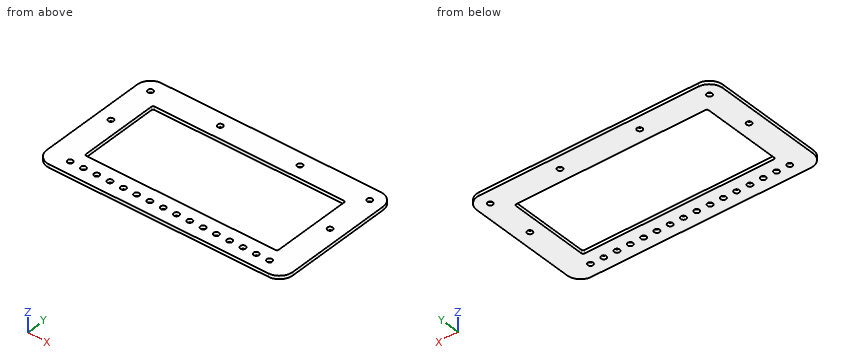
Autodesk Inventor part; units mm, degrees
ref_plane "YZ Plane" through (0, 0, 0) normal (1, 0, 0) x (0, 1, 0)
ref_plane "XZ Plane" through (0, 0, 0) normal (0, 1, 0) x (-1, 0, 0)
ref_plane "XY Plane" through (0, 0, 0) normal (0, 0, 1) x (1, 0, 0)
sketch "Sketch1" plane through (0, 0, 0) normal (0, 0, 1) x (1, 0, 0)
  line L0 (-92.075, -39.37) -> (92.075, -39.37)
  line L1 (92.075, -39.37) -> (92.075, 39.37)
  line L2 (92.075, 39.37) -> (-92.075, 39.37)
  line L3 (-92.075, 39.37) -> (-92.075, -39.37)
  line L4 (-92.075, -39.37) -> (92.075, 39.37) construction
  line L5 (92.075, -39.37) -> (-92.075, 39.37) construction
  line L6 (-117.475, 64.77) -> (117.475, 64.77)
  line L7 (117.475, 64.77) -> (117.475, -64.77)
  line L8 (117.475, -64.77) -> (-117.475, -64.77)
  line L9 (-117.475, -64.77) -> (-117.475, 64.77)
  point P0 (0, 0)
  dimension "d0" = 184.15
  dimension "d1" = 78.74
  dimension "d2" = 25.4
extrude "Plate1" add sketch "Sketch1" along normal mid plane 3.175
sketch "Sketch2" plane through (0, 0, 1.5875) normal (0, 0, 1) x (1, 0, 0)
  line L0 (-92.075, -39.37) -> (-92.075, 39.37) construction
  line L1 (-92.075, 39.37) -> (92.075, 39.37) construction
  line L2 (92.075, 39.37) -> (92.075, -39.37) construction
  line L3 (92.075, -39.37) -> (-92.075, -39.37) construction
  line L4 (104.775, 52.07) -> (-104.775, 52.07) construction
  line L5 (-104.775, 52.07) -> (-104.775, -52.07) construction
  line L6 (-104.775, -52.07) -> (104.775, -52.07) construction
  line L7 (104.775, -52.07) -> (104.775, 52.07) construction
  line L8 (0, 90.678) -> (0, -90.678) construction
  point P0 (0, 0)
  point P1 (-95.25, -52.07)
  point P2 (-82.55, -52.07)
  point P3 (-69.85, -52.07)
  point P4 (-57.15, -52.07)
  point P5 (-44.45, -52.07)
  point P6 (-31.75, -52.07)
  point P7 (-19.05, -52.07)
  point P8 (-6.35, -52.07)
  point P9 (6.35, -52.07)
  point P10 (19.05, -52.07)
  point P11 (31.75, -52.07)
  point P12 (44.45, -52.07)
  point P13 (57.15, -52.07)
  point P14 (69.85, -52.07)
  point P15 (82.55, -52.07)
  point P16 (95.25, -52.07)
  point P17 (-38.1, 52.07)
  point P18 (38.1, 52.07)
  point P19 (-104.775, 6.35)
  point P20 (104.775, 6.35)
  dimension "d4" = 12.7
  dimension "d16" = 12.7
  dimension "d21" = 9.525
  dimension "d22" = 9.525
  dimension "d23" = 66.675
  dimension "d24" = 66.675
  dimension "d25" = 76.2
  dimension "d26" = 45.72
  dimension "d28" = 45.72
hole "Hole1" at (-104.775, 52.07, 1.5875) at (104.775, 52.07, 1.5875) at (-95.25, -52.07, 1.5875) at (-82.55, -52.07, 1.5875) at (-69.85, -52.07, 1.5875) at (-57.15, -52.07, 1.5875) at (-44.45, -52.07, 1.5875) at (-31.75, -52.07, 1.5875) at (-19.05, -52.07, 1.5875) at (-6.35, -52.07, 1.5875) at (6.35, -52.07, 1.5875) at (19.05, -52.07, 1.5875) at (31.75, -52.07, 1.5875) at (44.45, -52.07, 1.5875) at (57.15, -52.07, 1.5875) at (69.85, -52.07, 1.5875) at (82.55, -52.07, 1.5875) at (95.25, -52.07, 1.5875) at (-38.1, 52.07, 1.5875) at (38.1, 52.07, 1.5875) at (-104.775, 6.35, 1.5875) at (104.775, 6.35, 1.5875) direction (0, 0, -1) diameter 5.1054 end through all
fillet "Corner Round1" radius 1.5875 4 edges at (-92.075, -39.37, 0) (-92.075, 39.37, 0) (92.075, 39.37, 0) (92.075, -39.37, 0)
fillet "Corner Round2" radius 12.7 4 edges at (-117.475, 64.77, 0) (117.475, 64.77, 0) (117.475, -64.77, 0) (-117.475, -64.77, 0)
equation "\"d34\" = Thickness"
equation "\"d3\" = Thickness"
equation "\"BendRadius\" = Thickness"
equation "\"BendReliefWidth\" = Thickness"
equation "\"BendReliefDepth\" = 0.5 * Thickness"
equation "\"CornerReliefSize\" = 4 * Thickness"
equation "\"MinimumRemnant\" = 2 * Thickness"
equation "\"TransitionRadius\" = BendRadius"
equation "\"JacobiRadiusSize\" = BendRadius"
equation "\"GapSize\" = Thickness"
properties part number "PLATE,MOUNT,BATTERY,TOP" material "Aluminum 3003-O"
The listing builds one solid part. Answer for the finished solid, in the listing's coordinates (mm). Coordinates: 2 decimals unless noted, no trailing zeros. Loops run counter-clockwise (first coordinate to the right, second up) from the corner with the lowest first, then second, coordinate; pieces in that order, holes last. Notation, with made-up numbers: (14, -29) -> (50, -29) arc R10 ccw to (50, -23) -> close; hole circle Ø6 at (17.5, 3). An arc over 180 degrees is marked (long way). Answer in a Markdown table with one row per item. Add a question column.
1. The part is cut by section D-D, the plane z = -0.7. Count the separate pieces of the cut face and the enclosed holes in it, then the cut area to 3 significant figures.
2. The part is cut by section B-B, the plane x = -38.1. Write down the section's boundary in (y, z).
3. The part is cut by section C-C, the plane x = 95.25. Write down the section's boundary in (y, z), then the cut area to 3 significant figures.
4. The part is cut by section A-A, the plane y = -6. Write down the section's boundary in (x, z) (1 decimal).
5. Consider line 1 (Y direction, x = 19.05, z = -0.15); line 2 (X direction, y = 21, z = -1.2) (3 decimals); line 3 (Y direction, x = 54.5, z = 0.3). Determine where each line is inside the solid, lowest interval first. Write a range as [from, to].
Answer below:
| question | item | result |
|---|---|---|
| 1 | separate pieces | 1 |
| 1 | enclosed holes | 23 |
| 1 | area | 15,300 mm2 |
| 2 | outline | (-64.77, -1.59) -> (-39.37, -1.59) -> (-39.37, 1.59) -> (-64.77, 1.59) -> close; (39.37, -1.59) -> (49.52, -1.59) -> (49.52, 1.59) -> (39.37, 1.59) -> close; (54.62, -1.59) -> (64.77, -1.59) -> (64.77, 1.59) -> (54.62, 1.59) -> close |
| 3 | outline | (-64.77, -1.59) -> (-54.62, -1.59) -> (-54.62, 1.59) -> (-64.77, 1.59) -> close; (-49.52, -1.59) -> (64.77, -1.59) -> (64.77, 1.59) -> (-49.52, 1.59) -> close |
| 3 | area | 395 mm2 |
| 4 | outline | (-117.5, -1.6) -> (-92.1, -1.6) -> (-92.1, 1.6) -> (-117.5, 1.6) -> close; (92.1, -1.6) -> (117.5, -1.6) -> (117.5, 1.6) -> (92.1, 1.6) -> close |
| 5 | line 1 | [-64.77, -54.62], [-49.52, -39.37], [39.37, 64.77] |
| 5 | line 2 | [-117.475, -92.075], [92.075, 117.475] |
| 5 | line 3 | [-64.77, -39.37], [39.37, 64.77] |
